from build123d import *

# Parameters (mm, degrees)
EXTRUDE_1_DEPTH     = 2
SKETCH_2_R          = 2
CUT_EXTRUDE_1_DEPTH = 2


with BuildPart() as part:
    # 草图1 → 凸台-拉伸1 (new body)
    with BuildSketch(Plane(origin=(0, 0, 0), x_dir=(1, 0, 0), z_dir=(0, 1, 0))):
        with BuildLine():
            Line((-75, 15), (75, 15))
            ThreePointArc((75, 15), (90, 0), (75, -15))
            Line((75, -15), (-75, -15))
            ThreePointArc((-75, -15), (-90, 0), (-75, 15))
        make_face()
    extrude(amount=EXTRUDE_1_DEPTH)

    # 草图2 → 切除-拉伸1 (cut)
    with BuildSketch(Plane(origin=(0, 2, 0), x_dir=(1, 0, 0), z_dir=(0, 1, 0))):
        with Locations(Location((-75, 5, 0), (0, 0, 270))):
            Circle(SKETCH_2_R)
        with Locations(Location((-75, -5, 0), (0, 0, 90))):
            Circle(SKETCH_2_R)
        with Locations(Location((75, -5, 0), (0, 0, 270))):
            Circle(SKETCH_2_R)
        with Locations(Location((75, 5, 0), (0, 0, 90))):
            Circle(SKETCH_2_R)
        with BuildLine():
            Line((-50, 6), (50, 6))
            ThreePointArc((50, 6), (56, 0), (50, -6))
            Line((50, -6), (-50, -6))
            ThreePointArc((-50, -6), (-56, 0), (-50, 6))
        make_face()
    extrude(amount=-CUT_EXTRUDE_1_DEPTH, mode=Mode.SUBTRACT)


solid = part.part
Can you work these out from the model? Positions are in its coordinate system, mm. A direction names the side the tool comes from. Give positions to 0.01 mm unless a question says otherwise; leave off trailing zeros. Order: outer loops, then holes, each group sorted by start corner. A loop starts at its lowest first (then second) coordinate and runs counter-clockwise, first axis right, second up. Notation, with made-up numbers: M -21.5,-0.5 L 9.5,-0.5 A27 ccw 9.5,30.5 Z; hole C 37,-39 d11. An arc over 180 degrees is marked long. One line per question, with ' | ' between items.
Item 1: Suppose I cut it at B-B, the plane y = 1.6. Write out the boundary of the cut face in (x, z).
Answer block:
outline: M -75,-15 L 75,-15 A15 ccw 75,15 L -75,15 A15 ccw Z; hole C -75,-5 d4; hole C -75,5 d4; hole M -50,-6 L 50,-6 A6 ccw 50,6 L -50,6 A6 ccw Z; hole C 75,-5 d4; hole C 75,5 d4
Item 2: I'm going to push a flat-ended pin straight in: pin 1 Ø3 at (x, z) = (75, 5) entering from +Y. Where does the tip first touch, or does it pass through?
Answer block:
pin 1: passes through
Item 3: Suppose I cut it at D-D, the plane z = -11.5. Write out the boundary of the cut face in (x, y), then the cut area to 3 significant figures.
Answer block:
outline: M -84.63,0 L 84.63,0 L 84.63,2 L -84.63,2 Z | area: 339 mm2
Item 4: For faces 1 (the face through (-90, 1, 0)), 2 (the face through (-56, 1, 0)), which set-ups out of +Z, -Z, +X, -X, +Y, -Y let a thin tool reach every point of the face, with its end or its side?
Answer block:
face 1: -X, +Y, -Y | face 2: +Y, -Y
Item 5: Please list where these lines run through material, in increasing order: L1, parallel to X at y = 1.2, z = -5; L2, parallel to Z at x = 9.5, y = 1.35; L3, parallel to Z at x = 74.5, y = 0.9.
Answer block:
L1: x = -89.14 to -77, -73 to -53.32, 53.32 to 73, 77 to 89.14 | L2: z = -15 to -6, 6 to 15 | L3: z = -15 to -6.94, -3.06 to 3.06, 6.94 to 15
Item 6: We'd pull the mould along X, two halves only. Please class faces 3 (the face through (90, 1, 0)), 4 (the face through (73, 1, -5)), 5 (the face through (-77, 1, 5)), 6 (the face through (1, 2, -7)): released by +X, released by -X, zero draft, split by the parting line, or undercut.
Answer block:
face 3: released by +X | face 4: undercut | face 5: undercut | face 6: zero draft
Item 7: Suppose I cut it at A-A, the plane x = -8.5. Write out the boundary of the cut face in (y, z), then the cut area to 3 significant figures.
Answer block:
outline: M 0,-15 L 2,-15 L 2,-6 L 0,-6 Z; M 0,6 L 2,6 L 2,15 L 0,15 Z | area: 36.0 mm2
Item 8: Suppose I cut it at C-C, the plane z = 9. Write out the boundary of the cut face in (x, y).
Answer block:
outline: M -87,0 L 87,0 L 87,2 L -87,2 Z
